Autodesk Inventor part; units mm, degrees
ref_plane "YZ Plane" through (0, 0, 0) normal (1, 0, 0) x (0, 1, 0)
ref_plane "XZ Plane" through (0, 0, 0) normal (0, 1, 0) x (-1, 0, 0)
ref_plane "XY Plane" through (0, 0, 0) normal (0, 0, 1) x (1, 0, 0)
sketch "Sketch1" plane through (0, 0, 0) normal (0, 0, 1) x (1, 0, 0)
  circle A0 centre (0, 0) radius 100
  dimension "d0" = 200
extrude "Extrusion1" add sketch "Sketch1" along normal blind 5
sketch "Sketch2" plane through (0, 0, 5) normal (0, 0, 1) x (1, 0, 0)
  circle A0 centre (0, 0) radius 87
  dimension "d3" = 174
extrude "Extrusion2" add sketch "Sketch2" along normal blind 5
sketch "Sketch3" plane through (0, 0, 10) normal (0, 0, 1) x (1, 0, 0)
  circle A0 centre (0, 0) radius 5
  dimension "d6" = 10
extrude "Extrusion3" cut sketch "Sketch3" against normal blind 10
sketch "Sketch4" plane through (0, 0, 10) normal (0, 0, 1) x (1, 0, 0)
  circle A0 centre (0, 0) radius 7.5
  circle A1 centre (0, 0) radius 5
  circle A2 centre (0, 0) radius 50
  dimension "d9" = 15
  dimension "d10" = 100
extrude "Extrusion4" cut sketch "Sketch4" against normal blind 7 contours A2
chamfer "Chamfer1" distance 5 distance2 40 1 edges at (-50, 0, 3) measured on face at (-30.4381, 39.6677, 7.6667)
sketch "Sketch10" plane through (0, 0, 0) normal (0, 0, -1) x (-1, 0, 0)
  circle A0 centre (0, 0) radius 100
  line L0 (0, -100) -> (0, -82.127)
  line L1 (0, -82.127) -> (20.7525, -82.127)
  line L2 (20.7525, -82.127) -> (-19.3985, -82.127)
  line L3 (-19.3985, -82.127) -> (-19.3985, -62.127)
  line L4 (-19.3985, -62.127) -> (20.7525, -62.127)
  line L5 (20.7525, -62.127) -> (20.7525, -82.127)
  dimension "d52" = 17.873
  dimension "d53" = 20.7525
  dimension "d54" = 40.151
  dimension "d55" = 20
extrude "Extrusion10" cut sketch "Sketch10" against normal blind 10 contours L2 L3 L4 L5 L1
properties part number "Rotating Plate"
The listing builds one solid part. Answer for the finished solid, in the listing's coordinates (mm). A direction names the side the tool comes from. Round coordinates to 2 decimals unless told otherwise and drop trailing zeros. Write each loop counter-clockwise with the first axis right and the second up, starting at its lowest first coordinate (ties: lowest second). Pieces come first, ordered by that corner, then holes. Notation, with made-up numbers: M 76,-15.75 L 98,-15.75 A19 cw 98,10.25 Z; hole C 14.5,48.5 d9. An arc over 180 degrees is marked long. Write each question's results on one line, items separated by ' | '. Start each with the question number.
Item 1: For a pull along X with two mould halves and no side action, classify faces 1 (the face through (47.69, 15.02, 9.01)), 2 (the face through (-11.33, -86.26, 7.46)), 3 (the face through (37, 40, 10)) as pulls with the +X half, pulls with the -X half, needs draft (parallel to the pull), parting line crosses it, or undercut.
Item 2: A cutting plane is placed at A-A on y = 0. Write down the section's boundary in (x, z).
Item 3: For faces 4 (the face through (2, -5, 10)), 5 (the face through (-75, 45, 5)), 6 (the face through (19.398, -72, 5)), determine the directions among +Z, -Z, +X, -X, +Y, -Y from which every point of the face is accessible in a straight line to the end or side of a thin tool.
Item 4: A cutting plane is placed at D-D on y = 55. Write down the section's boundary in (x, z).
Item 5: Flat-ended cylindrical pins translate along their axes: pin 1 Ø6 at (y, z) = (-76, 2) entering from +X; pin 2 Ø3 at (x, z) = (-3.5, 7.5) entering from -Y; pin 3 Ø3 at (y, z) = (-68, 4) entering from -X; pin 4 Ø4 at (x, y) = (-20.5, 63) entering from -Z. Find the tip coordinate at first contact, or state that the pin passes through.
Item 6: Straight lines are drawn through the part: L1, parallel to Y at x = 0, z = 2.75; L2, parallel to Y at x = 0, z = 8.55; L3, parallel to Z at x = -80, y = 40.5. For each, find the intervals that lie inside material, in ascending order. Write a range as [from, to].
Item 7: A cutting plane is placed at B-B on x = 0. Write down the section's boundary in (y, z).
Item 8: A cutting plane is placed at C-C on x = 60. Write down the section's boundary in (y, z).
Check sheet entries:
1) face 1: undercut | face 2: parting line crosses it | face 3: needs draft
2) outline: M -100,0 L -5,0 L -5,10 L -7.5,10 L -7.5,3 L -10,3 L -50,8 L -50,10 L -87,10 L -87,5 L -100,5 Z; M 5,0 L 100,0 L 100,5 L 87,5 L 87,10 L 50,10 L 50,8 L 10,3 L 7.5,3 L 7.5,10 L 5,10 Z
3) face 4: +Z, +X, -X, +Y, -Y | face 5: +Z | face 6: +Z, -Z
4) outline: M -83.52,0 L 83.52,0 L 83.52,5 L 67.41,5 L 67.41,10 L -67.41,10 L -67.41,5 L -83.52,5 Z
5) pin 1: x = 68.34 | pin 2: y = -86.98 | pin 3: x = -74.68 | pin 4: z = 0
6) L1: [-100, -82.13], [-62.13, -5], [5, 100] | L2: [-87, -82.13], [-62.13, -50], [-7.5, -5], [5, 7.5], [50, 87] | L3: [0, 5]
7) outline: M -100,0 L -82.13,0 L -82.13,10 L -87,10 L -87,5 L -100,5 Z; M -62.13,0 L -5,0 L -5,10 L -7.5,10 L -7.5,3 L -10,3 L -50,8 L -50,10 L -62.13,10 Z; M 5,0 L 100,0 L 100,5 L 87,5 L 87,10 L 50,10 L 50,8 L 10,3 L 7.5,3 L 7.5,10 L 5,10 Z
8) outline: M -80,0 L 80,0 L 80,5 L 63,5 L 63,10 L -63,10 L -63,5 L -80,5 Z
